Check sheet for the drawn part. Datum: minimum x, y, z corner. Units: mm. A direction names the side the tool comes from. Coordinates: 2 decimals unless noted, no trailing zeros. Write each loop counter-clockwise with the first axis right and the second up, starting at its lowest first coordinate (ties: lowest second). Pieces come first, ordered by that corner, then holes. Notation, with made-up numbers: (63, 40.25) -> (105, 40.25) arc R35 cw to (105, 77.25) -> close; hole circle Ø8 at (52, -7.75). An arc over 180 degrees is marked (long way). One line per question, with ' | ' between items.
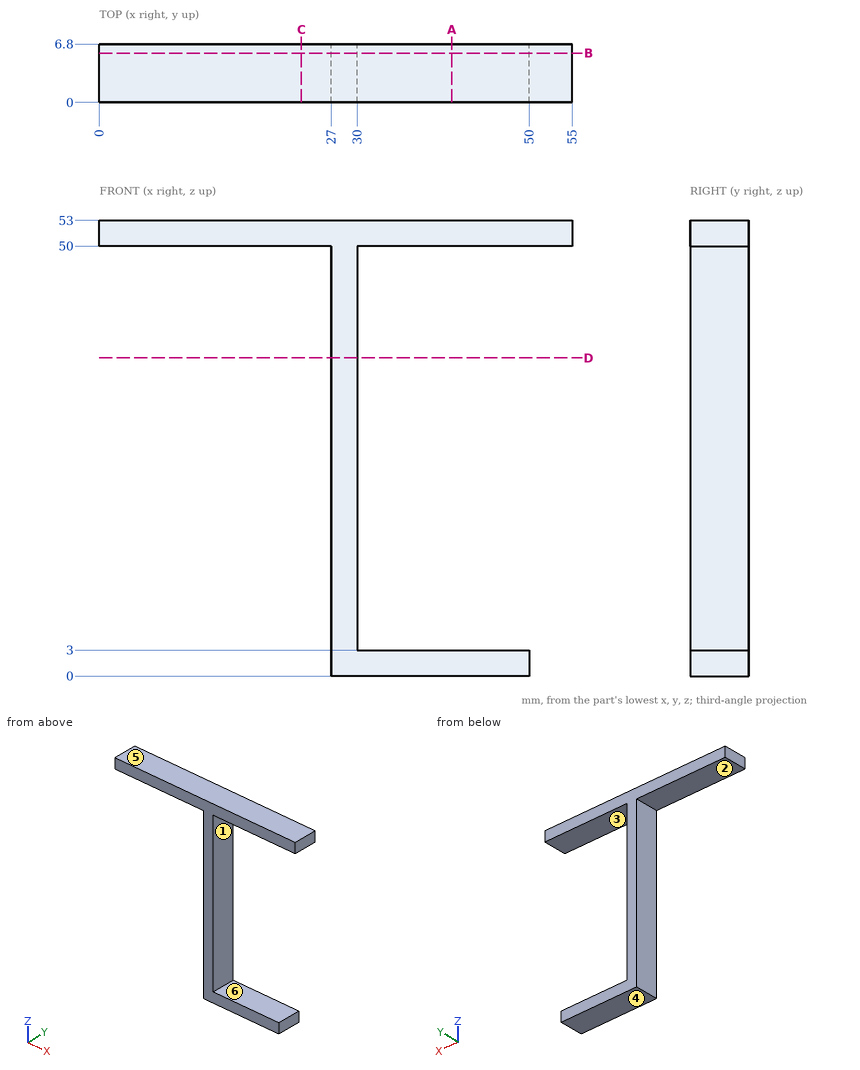
1. Go/stop test with flat-tipped pins: P1, Ø3.5, axis at y = 3, z = 38, coming from the +X side; P2, Ø2, axis at x = 12.5, y = 3.5, coming from the -Z side; P3, Ø3.5, axis at y = 3, z = 1, coming from the +X side. Record where each tip stops, or that it passes through.
Worked answers:
P1: x = 30 | P2: z = 50 | P3: x = 50
2. Cross-section at D-D on z = 37. Record the boundary of the cut face in (x, y), and give its area (3 significant figures).
Worked answers:
outline: (27, 0) -> (30, 0) -> (30, 6.8) -> (27, 6.8) -> close | area: 20.4 mm²
3. Material ranges on line 1 (Z direction, x = 35.5, y = 6); line 2 (X direction, y = 3.5, z = 45); line 3 (Z direction, x = 26.5, y = 5), recorded low to high. Write a range as from..to.
Worked answers:
line 1: 0..3, 50..53 | line 2: 27..30 | line 3: 50..53
4. Cross-section at B-B on y = 5.75. Record the boundary of the cut face in (x, z).
Worked answers:
outline: (0, 50) -> (27, 50) -> (27, 0) -> (50, 0) -> (50, 3) -> (30, 3) -> (30, 50) -> (55, 50) -> (55, 53) -> (0, 53) -> close
5. Cross-section at C-C on x = 23.5. Record the boundary of the cut face in (y, z).
Worked answers:
outline: (0, 50) -> (6.8, 50) -> (6.8, 53) -> (0, 53) -> close
6. Tool access check on the marked faces 1 and 2. Record the directions out of +Z, -Z, +X, -X, +Y, -Y that give a thin tool (end or side, any length) a straight path to the whole face; none if there is none.
Worked answers:
face 1: +X, +Y, -Y | face 2: -Z, -X, +Y, -Y
7. Mould release check, pull along Z, two halves, no side actions. Record for the marked faces 3, 4, 5 and 6: released by +Z, released by -Z, zero draft, split by the parting line, or undercut.
Worked answers:
face 3: undercut | face 4: released by -Z | face 5: released by +Z | face 6: undercut
8. Cross-section at A-A on x = 41. Record the boundary of the cut face in (y, z), and give its area (3 significant figures).
Worked answers:
outline: (0, 0) -> (6.8, 0) -> (6.8, 3) -> (0, 3) -> close; (0, 50) -> (6.8, 50) -> (6.8, 53) -> (0, 53) -> close | area: 40.8 mm²
